Source: three-view drawing plus pictorial views. Frame: mm from the lowest corner of the part. Coordinates: 2 decimals unless noted, no trailing zeros. Loops run counter-clockwise (first coordinate to the right, second up) from the corner with the lowest first, then second, coordinate; pieces in that order, holes last.
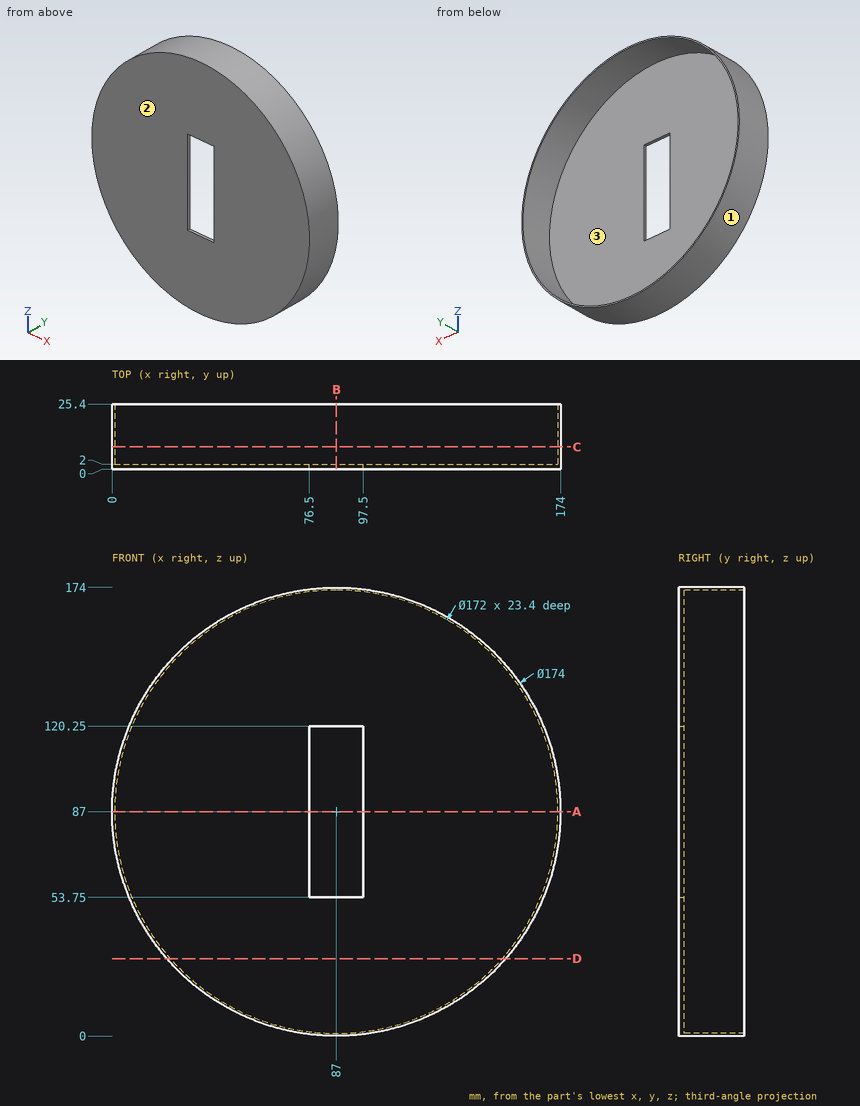
Q1. Draft query along Z for the marked faces 1, 2 and 3. Return one class per face: +Z half, -Z half, draft (parallel to the pull), parting line (faces both ways), or undercut.
Q2. Line query: line 1 along Z through (x, y) = (87, 15.5); line 2 along Y through (x, z) = (132.5, 153); line 3 along X through (y, z) = (9.5, 84). Output: solid intervals per line, ascending.
Q3. Section C-C, the plane y = 8.75. Return the cut outline in (x, z).
Q4. Contact query for flat-ended pins moving along their axis: pin 1 Ø10 at (x, z) = (30.5, 109.5) entering from +Y; pin 2 Ø0.6 at (x, y) = (91.5, 1) entering from -Z; pin 3 Ø1.6 at (y, z) = (1.5, 89) entering from -X. Output: stop coordinate, or through.
Q5. Section B-B, the plane x = 87. Return the cut outline in (y, z), plus the area to 3 significant figures.
Q6. Section A-A, the plane z = 87. Return the cut outline in (x, y), plus the area to 3 significant figures.
Q7. Section D-D, the plane z = 30. Return the cut outline in (x, y).
Derived:
1. face 1: parting line
1. face 2: draft
1. face 3: undercut
2. line 1: z = 0 to 1, 173 to 174
2. line 2: y = 0 to 2
2. line 3: x = 0.05 to 1.05, 172.95 to 173.95
3. outline: circle Ø174 at (87, 87); hole circle Ø172 at (87, 87)
4. pin 1: stops at y = 2
4. pin 2: stops at z = 0.1
4. pin 3: stops at x = 0.01
5. outline: (0, 0) - (25.4, 0) - (25.4, 1) - (2, 1) - (2, 53.75) - (0, 53.75) - close; (0, 120.25) - (2, 120.25) - (2, 173) - (25.4, 173) - (25.4, 174) - (0, 174) - close
5. area: 262 mm2
6. outline: (0, 0) - (76.5, 0) - (76.5, 2) - (1, 2) - (1, 25.4) - (0, 25.4) - close; (97.5, 0) - (174, 0) - (174, 25.4) - (173, 25.4) - (173, 2) - (97.5, 2) - close
6. area: 353 mm2
7. outline: (21.27, 0) - (152.73, 0) - (152.73, 25.4) - (151.4, 25.4) - (151.4, 2) - (22.6, 2) - (22.6, 25.4) - (21.27, 25.4) - close
